Build history of the part. All positions in model axes, mm. Face numbers are marked on the shaded views. Give positions to 0.01 mm unless a question says otherwise; leave off trailing zeros. Loops run counter-clockwise (first coordinate to the right, second up) from the corner with the lowest first, then second, coordinate; pieces in that order, holes last. Notation, with made-up numbers: (57.25, 35.25) -> (107.25, 35.25) arc R34 ccw to (107.25, 74.25) -> close; hole circle Ø11 at (36.25, -35). An arc over 180 degrees is marked (long way). Answer in a Markdown table with one row per item. Add a question column.
from build123d import *

# Parameters (mm, degrees)
SKETCH2_W           = 35
SKETCH2_H           = 2.5
SKETCH3_R           = 4
CUT_EXTRUDE1_DEPTH  = 3.5
CIRPATTERN1_COUNT   = 8
SKETCH11_R          = 6
SKETCH11_R_2        = 4
BOSS_EXTRUDE1_DEPTH = 2
FILLET1_R           = 1


with BuildPart() as part:
    # Sketch2 → Revolve1 (revolve)
    with BuildSketch(Plane.XY):
        with Locations((20.486722825, 7.5)):
            Rectangle(SKETCH2_W, SKETCH2_H)
    revolve(axis=Axis((2.986722825, 8.75, 0), (0, -1, 0)))

    # Sketch3 → Cut-Extrude1 (cut, through all)
    with BuildSketch(Plane(origin=(0, 8.75, 0), x_dir=(1, 0, 0), z_dir=(0, 1, 0))):
        with Locations((2.986722825, 0)):
            Circle(SKETCH3_R)
        with BuildLine():
            Line((11.953421812, 14.623553237), (5.81514995, 8.485281374))
            ThreePointArc((5.81514995, 8.485281374), (2.986722825, 7.313708499), (0.1582957, 8.485281374))
            Line((0.1582957, 8.485281374), (-5.979976162, 14.623553237))
            ThreePointArc((-5.979976162, 14.623553237), (-7.051976031, 18.338924141), (-4.478742954, 21.225381521))
            ThreePointArc((-4.478742954, 21.225381521), (2.986722825, 22.5), (10.452188604, 21.225381521))
            ThreePointArc((10.452188604, 21.225381521), (13.025421681, 18.338924141), (11.953421812, 14.623553237))
        make_face()
        with BuildLine():
            Line((11.953421812, -14.623553237), (5.81514995, -8.485281374))
            ThreePointArc((5.81514995, -8.485281374), (2.986722825, -7.313708499), (0.1582957, -8.485281374))
            Line((0.1582957, -8.485281374), (-5.979976162, -14.623553237))
            ThreePointArc((-5.979976162, -14.623553237), (-7.051976031, -18.338924141), (-4.478742954, -21.225381521))
            ThreePointArc((-4.478742954, -21.225381521), (2.986722825, -22.5), (10.452188604, -21.225381521))
            ThreePointArc((10.452188604, -21.225381521), (13.025421681, -18.338924141), (11.953421812, -14.623553237))
        make_face()
        with BuildLine():
            Line((-11.636830412, 8.966698987), (-5.498558549, 2.828427125))
            ThreePointArc((-5.498558549, 2.828427125), (-4.326985674, 0), (-5.498558549, -2.828427125))
            Line((-5.498558549, -2.828427125), (-11.636830412, -8.966698987))
            ThreePointArc((-11.636830412, -8.966698987), (-15.352201316, -10.038698856), (-18.238658696, -7.465465779))
            ThreePointArc((-18.238658696, -7.465465779), (-19.513277175, 0), (-18.238658696, 7.465465779))
            ThreePointArc((-18.238658696, 7.465465779), (-15.352201316, 10.038698856), (-11.636830412, 8.966698987))
        make_face()
        with BuildLine():
            Line((17.610276062, 8.966698987), (11.472004199, 2.828427125))
            ThreePointArc((11.472004199, 2.828427125), (10.300431324, 0), (11.472004199, -2.828427125))
            Line((11.472004199, -2.828427125), (17.610276062, -8.966698987))
            ThreePointArc((17.610276062, -8.966698987), (21.325646966, -10.038698856), (24.212104346, -7.465465779))
            ThreePointArc((24.212104346, -7.465465779), (25.486722825, 0), (24.212104346, 7.465465779))
            ThreePointArc((24.212104346, 7.465465779), (21.325646966, 10.038698856), (17.610276062, 8.966698987))
        make_face()
    extrude(amount=-CUT_EXTRUDE1_DEPTH, mode=Mode.SUBTRACT)

    # Sweep2: sweep along a path in Sketch9
    with BuildLine(Plane(origin=(0, 8.75, 0), x_dir=(1, 0, 0), z_dir=(0, 1, 0))) as sweep2_path:
        ThreePointArc((21.978484794, 18.991761969), (29.371276645, 10.5906167), (32.986722825, 0))
        ThreePointArc((32.986722825, 0), (33.102162214, -0.998284421), (33.182560833, -2))
    # Sketch1 → Sweep2 (sweep)
    with BuildSketch(Plane.XY):
        Polygon((34.11308378, 8.75), (33.294150753, 11), (32.679294897, 11), (31.86036187, 8.75), align=None)
    sweep2 = sweep(path=sweep2_path.line)

    # CirPattern1: Sweep2 ×8 about axis
    cirpattern1_axis = Axis((2.986722825, 6.25, 0), (0, 1, 0))
    for i in range(1, CIRPATTERN1_COUNT):
        add(sweep2.rotate(cirpattern1_axis, i * 360 / CIRPATTERN1_COUNT))

    # Sketch11 → Boss-Extrude1 (add)
    with BuildSketch(Plane(origin=(0, 8.75, 0), x_dir=(1, 0, 0), z_dir=(0, 1, 0))):
        with Locations((2.986722825, 0)):
            Circle(SKETCH11_R)
        with Locations((2.986722825, 0)):
            Circle(SKETCH11_R_2, mode=Mode.SUBTRACT)
    extrude(amount=BOSS_EXTRUDE1_DEPTH)

    # Fillet1
    fillet1_edges = [part.edges().sort_by_distance(p)[0] for p in [
        (-3.013277175, 8.75, 0),
    ]]
    fillet(fillet1_edges, radius=FILLET1_R)


solid = part.part
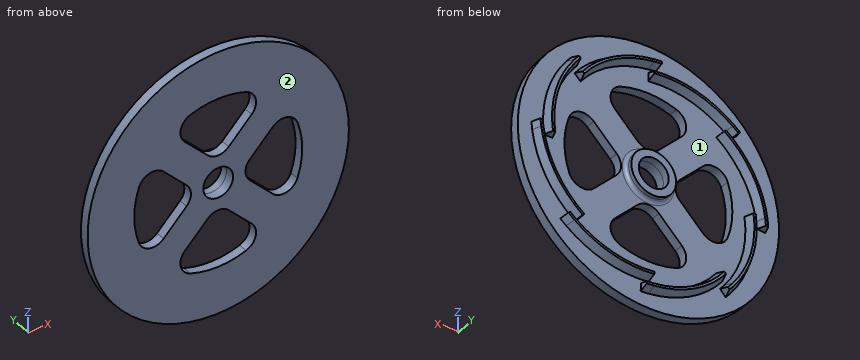
(1) Saw through at B-B, the plane x = 2. State how many separate pieces and enclosed holes the cut face has, then the cut area to 3 significant figures.
(2) Two-plate mould, pull along Z, no slides. Class the marked faces 1 and 2: released by +Z, released by -Z, zero draft, split by the parting line, or undercut.
(3) Flat gauge pins, fed straight in: pin 1 Ø1 at (x, y) = (22.5, 10) entering from +Z; pin 2 Ø1.5 at (x, y) = (-2.5, 7.5) entering from -Z; pin 3 Ø6 at (x, z) = (5.5, -2) entering from +Y. Where does each tip first touch, or does it go through?
(4) Saw through at A-A, the plane y = 7. List the corners of the cut face in (x, z) (3 decimals).
(5) Wall check: line 1 along Z through (x, y) = (2.5, 7.55); line 2 along Z through (x, y) = (12.5, 7.1); line 3 along Y through (x, z) = (29, 22.5). Give the ranges that are in metal, low to high. Write a range as from..to.
Worked answers:
| question | item | result |
|---|---|---|
| 1 | separate pieces | 4 |
| 1 | enclosed holes | 0 |
| 1 | area | 98.6 mm^2 |
| 2 | face 1 | undercut |
| 2 | face 2 | zero draft |
| 3 | pin 1 | z = 22.85 |
| 3 | pin 2 | z = -34.68 |
| 3 | pin 3 | y = 10.75 |
| 4 | outline | circle Ø70 at (2.987, 0); hole (-18.239, -7.465) arc R4 ccw to (-11.637, -8.967) -> (-5.499, -2.828) arc R4 ccw to (-5.499, 2.828) -> (-11.637, 8.967) arc R4 ccw to (-18.239, 7.465) arc R22.5 ccw to start; hole (-5.98, -14.624) arc R4 ccw to (-4.479, -21.225) arc R22.5 ccw to (10.452, -21.225) arc R4 ccw to (11.953, -14.624) -> (5.815, -8.485) arc R4 ccw to (0.158, -8.485) -> close; hole (-5.98, 14.624) -> (0.158, 8.485) arc R4 ccw to (5.815, 8.485) -> (11.953, 14.624) arc R4 ccw to (10.452, 21.225) arc R22.5 ccw to (-4.479, 21.225) arc R4 ccw to start; hole circle Ø8 at (2.987, 0); hole (11.472, -2.828) -> (17.61, -8.967) arc R4 ccw to (24.212, -7.465) arc R22.5 ccw to (24.212, 7.465) arc R4 ccw to (17.61, 8.967) -> (11.472, 2.828) arc R4 ccw to start |
| 5 | line 1 | -35..-22.49, -7.34..-3.97, 3.97..7.34, 22.49..35 |
| 5 | line 2 | -33.68..-19.6, -15.31..-3.86, 3.86..15.31, 19.6..33.68 |
| 5 | line 3 | 6.25..8.75 |
